Part print with two shaded views. Sizes in mm from the minimum x, y, z corner. A direction names the side the tool comes from. Round coordinates to 2 decimals unless told otherwise and drop trailing zeros. Order: outer loops, then holes, each group sorted by start corner. A loop starts at its lowest first (then second) coordinate and runs counter-clockwise, first axis right, second up. Notation, with made-up numbers: M 71.25,66.5 L 97.25,66.5 A17 cw 97.25,90.5 Z; hole C 50.5,32 d7. An arc over 180 degrees is marked long. Answer as a JSON object with one key per item and string values.
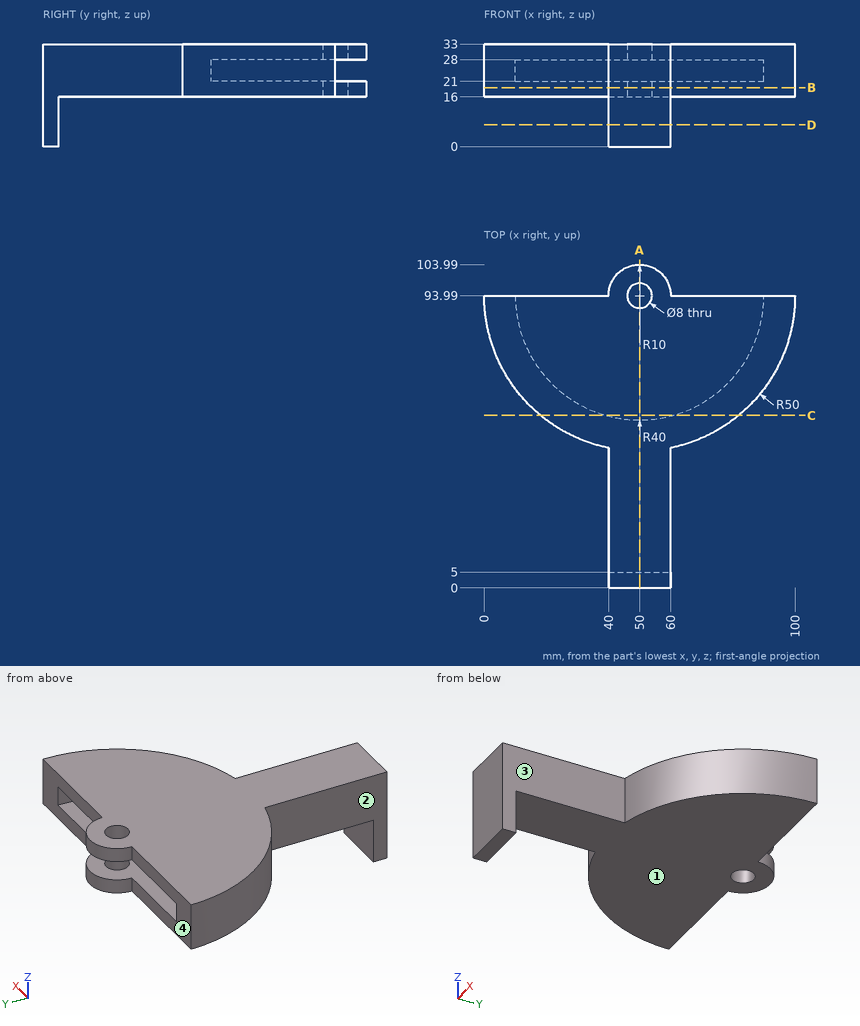
Item 1: Drop flat-ended pins along their axis: pin 1 Ø5 at (x, z) = (16.5, 28.5) entering from +Y; pin 2 Ø7 at (x, y) = (50, 93.99) entering from +Z; pin 3 Ø8 at (x, y) = (51, 43) entering from -Z; pin 4 Ø10 at (y, z) = (20.5, 16.5) entering from -X. Give the stop position or say it passes through.
Worked answers:
{"pin 1": "stops at y = 93.99", "pin 2": "passes through", "pin 3": "stops at z = 16", "pin 4": "stops at x = 40"}
Item 2: Saw through at D-D on z = 7. List the corners of the cut face in (x, y), and give its area (3 significant figures).
Worked answers:
{"outline": "M 40,0 L 60,0 L 60,5 L 40,5 Z", "area": "100 mm2"}
Item 3: Wall check: line 1 along Z through (x, y) = (40, 85.5); line 2 along Y through (x, z) = (50, 30.6); line 3 along Z through (x, y) = (53.5, 52). Give the ranges that are in metal, low to high. Write a range as [from, to].
Worked answers:
{"line 1": "z = [16, 21], [28, 33]", "line 2": "y = [0, 89.99], [97.99, 103.99]", "line 3": "z = [16, 33]"}
Item 4: 3-axis set-ups, long thin cutter, end or side, ignore diameter. For the marked faces 1, 2, 3 and 4: which of +Z, -Z, +X, -X, +Y, -Y reach the whole face in a straight line?
Worked answers:
{"face 1": "-Z, +X, -X, +Y", "face 2": "+Z, -Z, -X, -Y", "face 3": "+Z, -Z, +X, -Y", "face 4": "+Z, -Z, -X, +Y"}
Item 5: Saw through at A-A on x = 50. List the corners of the cut face in (y, z), and give its area (3 significant figures).
Worked answers:
{"outline": "M 0,0 L 5,0 L 5,16 L 89.99,16 L 89.99,21 L 53.99,21 L 53.99,28 L 89.99,28 L 89.99,33 L 0,33 Z; M 97.99,16 L 103.99,16 L 103.99,21 L 97.99,21 Z; M 97.99,28 L 103.99,28 L 103.99,33 L 97.99,33 Z", "area": "1,420 mm2"}
Item 6: Saw through at C-C on y = 55.5. List the corners of the cut face in (x, z), and give its area (3 significant figures).
Worked answers:
{"outline": "M 18.09,16 L 81.91,16 L 81.91,33 L 18.09,33 Z; hole M 39.11,21 L 60.89,21 L 60.89,28 L 39.11,28 Z", "area": "933 mm2"}
Item 7: Saw through at B-B on z = 19. List the corners of the cut face in (x, y).
Worked answers:
{"outline": "M 0,93.99 A50 ccw 40,45 L 40,0 L 60,0 L 60,45 A50 ccw 100,93.99 L 60,93.99 A10 ccw 40,93.99 Z; hole C 50,93.99 d8"}
